The listing builds one solid part. Answer for the finished solid, in the listing's coordinates (mm). Face numbers are marked on the shaded views. Coordinates: 2 decimals unless noted, no trailing zeros. Loops run counter-clockwise (first coordinate to the right, second up) from the corner with the lowest first, then second, coordinate; pieces in that order, holes last. Notation, with made-up numbers: (-21.5, 41.25) -> (-1.5, 41.25) arc R21 cw to (-1.5, 50.25) -> close; hole circle Ø2 at (63.5, 31.5). An arc over 180 degrees is marked (long way). Answer in a Markdown table with one row per item.
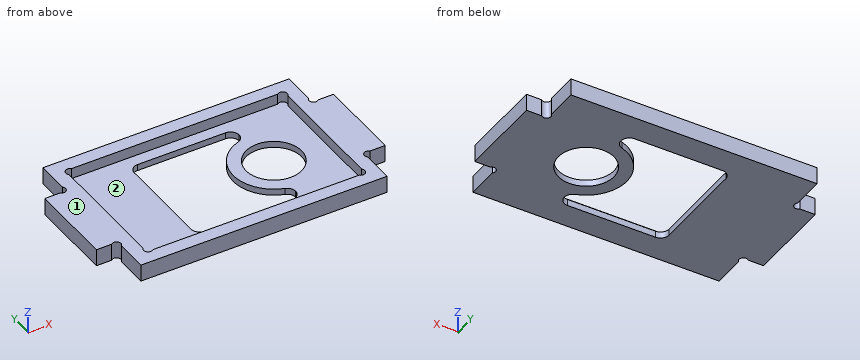
Autodesk Inventor part; units mm, degrees
ref_plane "YZ Plane" through (0, 0, 0) normal (1, 0, 0) x (0, 1, 0)
ref_plane "XZ Plane" through (0, 0, 0) normal (0, 1, 0) x (-1, 0, 0)
ref_plane "XY Plane" through (0, 0, 0) normal (0, 0, 1) x (1, 0, 0)
sketch "スケッチ1" plane through (0, 0, 0) normal (0, 0, 1) x (1, 0, 0)
  line L0 (12, 16) -> (-29, 16) construction
  line L1 (-31, 14) -> (-31, -14) construction
  line L2 (-29, -16) -> (12, -16) construction
  line L3 (12, -16) -> (12, 16) construction
  line L4 (12, 16) -> (-31, -16) construction
  line L5 (-31, 16) -> (12, -16) construction
  line L6 (12, 0) -> (-31, 0) construction
  circle A0 centre (0, 0) radius 10.5 construction
  arc A1 (12, 10.583) -> (0, 16) centre (0, 0) ccw construction
  line L7 (-39.5, 14.4) -> (-39.5, -14.4) construction
  arc A2 (-29, 16) -> (-31, 14) centre (-29, 14) ccw construction
  arc A3 (-31, -14) -> (-29, -16) centre (-29, -14) ccw construction
  line L8 (-39.5, 14.4) -> (-30.9596, 14.4) construction
  line L9 (-39.5, -14.4) -> (-30.9596, -14.4) construction
  line L10 (-1, 13.5) -> (-28, 13.5) construction
  line L11 (-28, 13.5) -> (-28, -13.5) construction
  line L12 (-28, -13.5) -> (-1, -13.5) construction
  line L13 (-1, -13.5) -> (-1, 13.5) construction
  line L14 (-1, 13.5) -> (-28, -13.5) construction
  line L15 (-28, 13.5) -> (-1, -13.5) construction
  circle A4 centre (-1, 13.5) radius 1.35 construction
  circle A5 centre (-28, 13.5) radius 1.35 construction
  circle A6 centre (-1, -13.5) radius 1.35 construction
  circle A7 centre (-28, -13.5) radius 1.35 construction
  arc A8 (0, -16) -> (12, -10.583) centre (0, 0) ccw construction
  line L16 (11.9, 15.8) -> (11.9, 14.3151) construction
  line L17 (11.9, 15.8) -> (10.4151, 15.8) construction
  line L18 (-39.225, 15.8) -> (-39.225, 14.3151) construction
  arc A9 (-37.7401, 15.8) -> (-39.225, 14.3151) centre (-38.4825, 15.0575) ccw
  line L19 (11.9, -15.8) -> (10.4151, -15.8) construction
  arc A10 (-39.225, -14.3151) -> (-37.7401, -15.8) centre (-38.4825, -15.0575) ccw
  line L20 (-42.5, 19) -> (15, 19)
  line L21 (15, 19) -> (15, -19) construction
  line L22 (15, -19) -> (-42.5, -19)
  line L23 (-42.5, -19) -> (-42.5, 19) construction
  line L24 (-42.5, 19) -> (15, -19) construction
  line L25 (15, 19) -> (-42.5, -19) construction
  line L26 (15, 10) -> (16.4849, 10) construction
  line L27 (20, 10) -> (20, -10)
  line L28 (15, -10) -> (16.4849, -10) construction
  arc A11 (15, 11.4849) -> (16.4849, 10) centre (15.7425, 10.7425) ccw
  arc A12 (16.4849, -10) -> (15, -11.4849) centre (15.7425, -10.7425) ccw
  line L29 (-13.75, 19) -> (-13.75, -19) construction
  line L30 (15, 11.4849) -> (15, 19)
  line L31 (15, -11.4849) -> (15, -19)
  line L32 (-42.5, 10) -> (-43.9849, 10) construction
  line L33 (-47.5, 10) -> (-47.5, -10)
  line L34 (-42.5, -10) -> (-43.9849, -10) construction
  arc A13 (-43.9849, 10) -> (-42.5, 11.4849) centre (-43.2425, 10.7425) ccw
  arc A14 (-42.5, -11.4849) -> (-43.9849, -10) centre (-43.2425, -10.7425) ccw
  line L35 (-42.5, 11.4849) -> (-42.5, 19)
  line L36 (-42.5, -11.4849) -> (-42.5, -19)
  circle A15 centre (0, 0) radius 6 construction
  circle A16 centre (0, 0) radius 6.5
  line L37 (-3.5, 13) -> (-24, 13)
  line L38 (-26, 11) -> (-26, -11)
  line L39 (-3.5, -13) -> (-24, -13)
  arc A17 (-24, 13) -> (-26, 11) centre (-24, 11) ccw
  arc A18 (-26, -11) -> (-24, -13) centre (-24, -11) ccw
  line L40 (-1.5, 11) -> (-1.5, 10.9545)
  arc A19 (-2.8913, 9.0493) -> (-2.8913, -9.0493) centre (0, 0) ccw
  line L41 (-1.5, -10.9545) -> (-1.5, -11)
  arc A20 (-1.5, 11) -> (-3.5, 13) centre (-3.5, 11) ccw
  arc A21 (-3.5, -13) -> (-1.5, -11) centre (-3.5, -11) ccw
  arc A22 (-1.5, -10.9545) -> (-2.8913, -9.0493) centre (-3.5, -10.9545) ccw
  arc A23 (-2.8913, 9.0493) -> (-1.5, 10.9545) centre (-3.5, 10.9545) ccw
  arc A24 (11.9, 14.3151) -> (10.4151, 15.8) centre (11.1575, 15.0575) ccw
  arc A25 (10.4151, -15.8) -> (11.9, -14.3151) centre (11.1575, -15.0575) ccw
  line L42 (10.4151, 15.8) -> (-37.7401, 15.8)
  line L43 (11.9, 14.3151) -> (11.9, -14.3151)
  line L44 (10.4151, -15.8) -> (-37.7401, -15.8)
  line L45 (11.9, -14.3151) -> (11.9, -15.8) construction
  line L46 (-37.7401, -15.8) -> (-39.225, -15.8) construction
  line L47 (-39.225, -14.3151) -> (-39.225, -15.8) construction
  line L48 (-37.7401, 15.8) -> (-39.225, 15.8) construction
  line L49 (-39.225, 14.3151) -> (-39.225, -14.3151)
  line L50 (16.4849, 10) -> (20, 10)
  line L51 (16.4849, -10) -> (20, -10)
  line L52 (-43.9849, -10) -> (-47.5, -10)
  line L53 (-43.9849, 10) -> (-47.5, 10)
  point P0 (-9.5, 0)
  point P1 (-14.5, 0)
  point P2 (-13.75, 0)
  point P3 (-39.225, -14.3151)
  point P4 (-43.9849, -10)
  point P5 (-1.5, 13)
  point P6 (-26, 13)
  point P7 (-1.5, -13)
  point P8 (-26, -13)
  point P9 (-1.5, -13)
  point P10 (-1.5, 13)
  point P11 (-1.5, 9.3808)
  point P12 (-1.5, -9.3808)
  point P13 (11.9, -14.3151)
  point P14 (10.4151, -15.8)
  dimension "d0" = 43
  dimension "d1" = 32
  dimension "d2" = 21
  dimension "d3" = 16
  dimension "d4" = 9.5
  dimension "d5" = 28.8
  dimension "d7" = 2
  dimension "d8" = 8.5
  dimension "d9" = 27
  dimension "d10" = 27
  dimension "d11" = 8.5
  dimension "d12" = 2.7
  dimension "d13" = 2.7
  dimension "d23" = 3
  dimension "d24" = 3
  dimension "d26" = 5
  dimension "d27" = 20
  dimension "d29" = 1.05
  dimension "d34" = 12
  dimension "d35" = 13
  dimension "d36" = 38
  dimension "d39" = 5
  dimension "d40" = 2
  dimension "d43" = 3
  dimension "d44" = 3
  dimension "d45" = 1.5
  dimension "d46" = 2
  dimension "d47" = 2
  dimension "d54" = 51.125
  dimension "d55" = 0.1
  dimension "d57" = 31.6
  dimension "d58" = 2.1
  dimension "d59" = 2.1
extrude "押し出し1" add sketch "スケッチ1" along normal blind 4 contours L20 L30 A11 L50 L27 L51 A12 L31 L22 L36 A14 L52 L33 L53 A13 L35
extrude "押し出し2" add sketch "スケッチ1" along normal blind 1.5 contours L42 A24 L43 A25 L44 A10 L49 A9
equation "\"d13\" = d12"
equation "\"d24\" = d23"
equation "\"d29\" = d17"
equation "\"d39\" = d38"
equation "\"d38\" = d37"
properties part number "Trunk_servo_bottom_frame" material "アルミニウム 2014-T4"
Item 1: A cutting plane is placed at C-C, the plane x = 0. Determine the outline of the cut face in (y, z).
Findings below:
| item | result |
|---|---|
| outline | (-19, 0) -> (-6.5, 0) -> (-6.5, 1.5) -> (-15.8, 1.5) -> (-15.8, 4) -> (-19, 4) -> close; (6.5, 0) -> (19, 0) -> (19, 4) -> (15.8, 4) -> (15.8, 1.5) -> (6.5, 1.5) -> close |
Item 2: Flat-ended cylindrical pins translate along their axes: pin 1 Ø2 at (y, z) = (16.5, 2) entering from +X; pin 2 Ø10 at (x, y) = (-12, 1) entering from -Z; pin 3 Ø1 at (x, y) = (-6.5, -4.5) entering from +Z; pin 4 Ø1.2 at (y, z) = (-17, 3) entering from -X. Find the tip coordinate at first contact, or state that the pin passes through.
Findings below:
| item | result |
|---|---|
| pin 1 | stops at x = 15 |
| pin 2 | stops at z = 0 |
| pin 3 | stops at z = 1.5 |
| pin 4 | stops at x = -42.5 |
Item 3: A cutting plane is placed at B-B, the plane y = 0. Determine the outline of the cut face in (x, z) (3 decimals).
Findings below:
| item | result |
|---|---|
| outline | (-47.5, 0) -> (-26, 0) -> (-26, 1.5) -> (-39.225, 1.5) -> (-39.225, 4) -> (-47.5, 4) -> close; (-9.5, 0) -> (-6.5, 0) -> (-6.5, 1.5) -> (-9.5, 1.5) -> close; (6.5, 0) -> (20, 0) -> (20, 4) -> (11.9, 4) -> (11.9, 1.5) -> (6.5, 1.5) -> close |
Item 4: A cutting plane is placed at A-A, the plane z = 2.1. Determine the outline of the cut face in (x, y) (1 decimal), plus the area to 3 significant figures.
Findings below:
| item | result |
|---|---|
| outline | (-47.5, -10) -> (-44, -10) arc R1 cw to (-42.5, -11.5) -> (-42.5, -19) -> (15, -19) -> (15, -11.5) arc R1 cw to (16.5, -10) -> (20, -10) -> (20, 10) -> (16.5, 10) arc R1 cw to (15, 11.5) -> (15, 19) -> (-42.5, 19) -> (-42.5, 11.5) arc R1 cw to (-44, 10) -> (-47.5, 10) -> close; hole (-39.2, -14.3) arc R1 ccw to (-37.7, -15.8) -> (10.4, -15.8) arc R1 ccw to (11.9, -14.3) -> (11.9, 14.3) arc R1 ccw to (10.4, 15.8) -> (-37.7, 15.8) arc R1 ccw to (-39.2, 14.3) -> close |
| area | 764 mm2 |
Item 5: Find the intervals of material crossed by probe 1 along Y at (x, z) = (-15, 3.15); probe 2 along X at (y, z) = (9, 1.7) (3 decimals); probe 3 along Y at (x, z) = (0, 0.3), in increasing order.
Findings below:
| item | result |
|---|---|
| probe 1 | y = -19 to -15.8, 15.8 to 19 |
| probe 2 | x = -47.5 to -39.225, 11.9 to 20 |
| probe 3 | y = -19 to -6.5, 6.5 to 19 |
Item 6: A cutting plane is placed at D-D, the plane x = -29. Determine the outline of the cut face in (y, z).
Findings below:
| item | result |
|---|---|
| outline | (-19, 0) -> (19, 0) -> (19, 4) -> (15.8, 4) -> (15.8, 1.5) -> (-15.8, 1.5) -> (-15.8, 4) -> (-19, 4) -> close |
Item 7: Determine the mould class of the marked faces 1 and 2 for opening direction X: +X half, -X half, draft (parallel to the pull), parting line (faces both ways), or undercut.
Findings below:
| item | result |
|---|---|
| face 1 | draft |
| face 2 | undercut |
